Geometry: final body of the model. Coordinates: model frame, mm. A direction names the side the tool comes from. Give positions to 0.01 mm unless a question says otherwise; leave off trailing zeros. Loops run counter-clockwise (first coordinate to the right, second up) from the corner with the lowest first, then second, coordinate; pieces in that order, holes last. Notation, with made-up numbers: (55.5, 18) - (104.5, 18) arc R22 ccw to (104.5, 35) - close; hole circle Ø5 at (11, 40.25). An arc over 180 degrees is marked (long way). Use CSV: the item, a comma, the result in double quotes. Start each with the question number.
```python
from build123d import *

# Parameters (mm, degrees)
F0_R          = 1.75
F1_DEPTH      = 3
F3_DEPTH      = 1.5
F3_DEPTH_BACK = 4.5
F4_T1_DEPTH   = 35.8553046099
F4_T3_DEPTH   = 35
F5_R          = 3
F6_DEPTH      = 1.5


# Not quite as in the source:
# - a fillet or chamfer that OpenCascade refuses, or shapes differently, is made with other operations: its cross-section is extruded or revolved along the edge and cut away or added
# - a feature names something its author has since deleted; it is built from what else it names


with BuildPart() as f1:
    # F0 (on Top) → F1 (new body)
    with BuildSketch(Plane.XY):
        with BuildLine():
            Line((-5.5846913819, -42.1934081889), (5.5801667099, -42.1934081889))
            ThreePointArc((5.5801667099, -42.1934081889), (6.2571567858, -41.9294003336), (6.5766854657, -41.2767770629))
            Line((6.5766854657, -41.2767770629), (10.8664863973, 9.9997591089))
            Line((10.8664863973, 9.9997591089), (12.9481358013, 16.1793168214))
            ThreePointArc((12.9481358013, 16.1793168214), (13.3997566467, 18.3576501573), (13.4874998392, 20.5805758517))
            Line((13.4874998392, 20.5805758517), (13.4943094486, 20.6080656878))
            ThreePointArc((13.4943094486, 20.6080656878), (13.4214184301, 22.4544852439), (13.0970679667, 24.2736540252))
            Line((13.0970679667, 24.2736540252), (10.3058793621, 33.9058264779))
            Line((10.3058793621, 33.9058264779), (9.4093267365, 36.9997591089))
            Line((9.4093267365, 36.9997591089), (4.9829727946, 36.9997591089))
            Line((4.9829727946, 36.9997591089), (-5.25, 36.9997591089))
            Line((-5.25, 36.9997591089), (-10.5906732635, 36.9997591089))
            Line((-10.5906732635, 36.9997591089), (-10.7942270682, 35.9658364889))
            Line((-10.7942270682, 35.9658364889), (-13.0926909538, 24.2911158576))
            Line((-13.0926909538, 24.2911158576), (-13.3631447598, 22.9173841889))
            ThreePointArc((-13.3631447598, 22.9173841889), (-13.4782769531, 21.765539271), (-13.4943094486, 20.6080656878))
            Line((-13.4943094486, 20.6080656878), (-13.4876078419, 20.5780624058))
            ThreePointArc((-13.4876078419, 20.5780624058), (-13.3996035826, 18.3564016222), (-12.9481358013, 16.1793168214))
            Line((-12.9481358013, 16.1793168214), (-11.1248120452, 9.9997591089))
            Line((-11.1248120452, 9.9997591089), (-6.5807885254, -41.281671889))
            ThreePointArc((-6.5807885254, -41.281671889), (-6.259871469, -41.9310611222), (-5.5846913819, -42.1934081889))
        make_face()
        with Locations((-5.25, 2.9997591089)):
            Circle(F0_R, mode=Mode.SUBTRACT)
        with Locations((5.25, 2.9997591089)):
            Circle(F0_R, mode=Mode.SUBTRACT)
        with BuildLine():
            ThreePointArc((-13.0926909538, 24.2911158576), (-13.2457387677, 23.6077585201), (-13.3631447598, 22.9173841889))
            Line((-13.3631447598, 22.9173841889), (-13.0926909538, 24.2911158576))
        make_face()
    extrude(amount=F1_DEPTH)

    # F2 (on face) → F3 (join, two sides)
    with BuildSketch(Plane.XY.offset(3)) as f3_sk:
        Polygon((9.4093267365, 36.9997591089), (-10.5906732635, 36.9997591089), (-11.7496770502, 31.1127641011), (11.1152465029, 31.1127641011), align=None)
    extrude(amount=F3_DEPTH)
    extrude(f3_sk.sketch, amount=-F3_DEPTH_BACK)

    # F4: fillet of radius 3 on 4 edges, made by hand

    # F4_s2 → F4_t1 (cut)
    with BuildSketch(Plane.YZ.offset(-18.2448675786)):
        with BuildLine():
            ThreePointArc((33.7108403124, 4.5), (32.2108403124, 4.0980762114), (31.1127641011, 3))
            Line((31.1127641011, 3), (31.1127641011, 4.5))
            Line((31.1127641011, 4.5), (33.7108403124, 4.5))
        make_face()
        with BuildLine():
            ThreePointArc((31.1127641011, 0), (32.2108403124, -1.0980762114), (33.7108403124, -1.5))
            Line((33.7108403124, -1.5), (31.1127641011, -1.5))
            Line((31.1127641011, -1.5), (31.1127641011, 0))
        make_face()
    extrude(amount=F4_T1_DEPTH, mode=Mode.SUBTRACT)

    # F4_s4 → F4_t3 (cut)
    with BuildSketch(Plane.YZ.offset(-18.0906732635)):
        with BuildLine():
            ThreePointArc((36.9997591089, 1.5), (36.1210794525, 3.6213203436), (33.9997591089, 4.5))
            Line((33.9997591089, 4.5), (36.9997591089, 4.5))
            Line((36.9997591089, 4.5), (36.9997591089, 1.5))
        make_face()
        with BuildLine():
            ThreePointArc((33.9997591089, -1.5), (36.1210794525, -0.6213203436), (36.9997591089, 1.5))
            Line((36.9997591089, 1.5), (36.9997591089, -1.5))
            Line((36.9997591089, -1.5), (33.9997591089, -1.5))
        make_face()
    extrude(amount=F4_T3_DEPTH, mode=Mode.SUBTRACT)

    # F5 (on face) → F6 (cut)
    with BuildSketch(Plane.XY.offset(3)):
        with Locations((-5.25, 2.9997591089)):
            Circle(F5_R)
        with Locations((5.25, 2.9997591089)):
            Circle(F5_R)
    extrude(amount=-F6_DEPTH, mode=Mode.SUBTRACT)


solid = f1.part
```
Item 1: Mould query, pull axis X, two halves, no side actions, for faces 5 (the cylindrical face through (-0.48, 32.23, 4.11)), 6 (the flat face through (7, 2, 1.5)), 7 (the flat face through (-12.05, 13.13, 1.48)). Classes: pulls with the +X half, pulls with the -X half, needs draft (parallel to the pull), parting line crosses it, or undercut.
Item 2: Section D-D (y = -35.5). Output: boundary loops of the cut face in (x, z), plus the area to 3 significant figures.
Item 3: Section C-C (x = -9). Output: boundary loops of the cut face in (y, z), plus the area to 3 significant figures.
Item 4: Section B-B (y = 32). Output: boundary loops of the cut face in (x, z) (3 decimals), plus the area to 3 significant figures.
Item 5: Ray query, probe 1 along Y at (x, z) = (5.25, 1.2); probe 2 along Z at (x, y) = (9, -9); probe 3 along Y at (x, z) = (-5.25, 0.7). Return the intervals inside material, ascending.
Item 6: Reachability of faces 1 (the cylindrical face through (8.02, 1.85, 2.26)), 2 (the flat face through (0, 3, 3)), 3 (the flat face through (0, 3, 0)), 4 (the cylindrical face through (3.5, 3.08, 0.74)) from +Z, -Z, +X, -X, +Y, -Y: full face, straight path, thin tool, end or side. Return the list, or none.
Item 7: Pin query (flat end, axial travel): pin 1 Ø3 at (x, y) = (-6, 2) entering from +Z; pin 2 Ø4 at (x, y) = (5.25, 3) entering from -Z; pin 3 Ø6.5 at (x, y) = (6, 2.5) entering from +Z. Return the tip coordinate at first contact, or that it passes through.
Item 8: Section A-A (x = 1.25). Output: boundary loops of the cut face in (y, z).
Outcome:
1,face 5,"needs draft"
1,face 6,"undercut"
1,face 7,"pulls with the -X half"
2,outline,"(-7.09, 0) - (7.06, 0) - (7.06, 3) - (-7.09, 3) - close"
2,area,"42.5 mm2"
3,outline,"(-13.98, 0) - (31.11, 0) arc R3 ccw to (33.71, -1.5) - (34, -1.5) arc R3 ccw to (34, 4.5) - (33.71, 4.5) arc R3 ccw to (31.11, 3) - (-13.98, 3) - close"
3,area,"164 mm2"
4,outline,"(-11.575, -0.964) - (10.858, -0.964) - (10.858, 3.964) - (-11.575, 3.964) - close"
4,area,"111 mm2"
5,probe 1,"y = -42.19 to 1.25, 4.75 to 36.98"
5,probe 2,"z = 0 to 3"
5,probe 3,"y = -42.19 to 1.25, 4.75 to 36.89"
6,face 1,"+Z"
6,face 2,"+Z, +X, -X, -Y"
6,face 3,"-Z, +X, -X, -Y"
6,face 4,"+Z, -Z"
7,pin 1,"stops at z = 1.5"
7,pin 2,"stops at z = 0"
7,pin 3,"stops at z = 3"
8,outline,"(-42.19, 0) - (31.11, 0) arc R3 ccw to (33.71, -1.5) - (34, -1.5) arc R3 ccw to (34, 4.5) - (33.71, 4.5) arc R3 ccw to (31.11, 3) - (-42.19, 3) - close"
